Can you work these out from the model? Positions are in its coordinate system, mm. Round coordinates to 2 decimals unless told otherwise and drop trailing zeros. Loops run counter-clockwise (first coordinate to the right, second up) from the corner with the lowest first, then second, coordinate; pieces in that order, holes last. Notation, with made-up numbers: M 64,40.25 L 87,40.25 A22 cw 87,58.25 Z; hole C -19,78 d3. An arc over 180 degrees is marked long. Use a Markdown table: item, result. Add a question column.
```python
from build123d import *

# Parameters (mm, degrees)
SKETCH004_W  = 5.019769
SKETCH004_H  = 1.561025
PAD002_DEPTH = 1
PAD_DEPTH    = 0.5
PAD001_DEPTH = 0.5
PAD003_DEPTH = 0.5
PAD004_DEPTH = 0.5


with BuildPart() as part:
    # Sketch004 → Pad002 (new body)
    with BuildSketch(Plane.XZ.offset(1.25)):
        with Locations((1.436677, 3.083954)):
            Rectangle(SKETCH004_W, SKETCH004_H)
    extrude(amount=PAD002_DEPTH)

    # Sketch → Pad (join)
    with BuildSketch(Plane.YZ.offset(-0.75)):
        Polygon((-1.5, 3), (0.5, 3), (0.5, 17.5), (0, 17.5), (0, 3.5), (-1.5, 3.5), align=None)
    extrude(amount=PAD_DEPTH)

    # Sketch001 → Pad001 (join)
    with BuildSketch(Plane.YZ.offset(0.5)):
        Polygon((-1.5, 3), (0.5, 3), (0.5, 17.5), (0, 17.5), (0, 3.5), (-1.5, 3.5), align=None)
    extrude(amount=PAD001_DEPTH)

    # Sketch002 → Pad003 (join)
    with BuildSketch(Plane.YZ.offset(1.75)):
        Polygon((-1.5, 3), (0.5, 3), (0.5, 17.5), (0, 17.5), (0, 3.5), (-1.5, 3.5), align=None)
    extrude(amount=PAD003_DEPTH)

    # Sketch003 → Pad004 (join)
    with BuildSketch(Plane.YZ.offset(3)):
        Polygon((-1.5, 3), (0.5, 3), (0.5, 17.5), (0, 17.5), (0, 3.5), (-1.5, 3.5), align=None)
    extrude(amount=PAD004_DEPTH)


solid = part.part
```
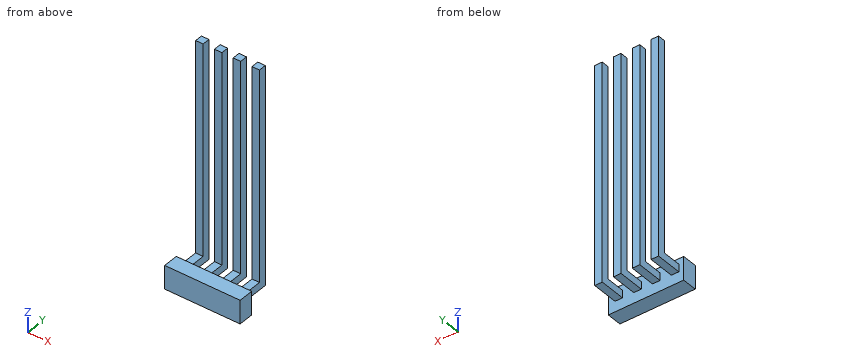
(1) I'm going to push flat-ended pins straight in: pin 1 (0.5 mm diameter, centred on y = 0, z = 11.5, fed in from +X); pin 2 (1 mm diameter, centred on x = 1.5, y = -0.5, fed in from +Z); pin 3 (0.6 mm diameter, centred on x = 1, y = -0.5, fed in from -Z). Where does each tip first touch, or does it pass through?
(2) Suppose I cut it at B-B on y = -0.25. List the corners of the cut face in (x, z) for me.
(3) Suppose I cut it at C-C on x = 0.7. List the corners of the cut face in (y, z) for me, and give its area (3 significant figures).
(4) Suppose I cut it at D-D on y = -1.8. List the corners of the cut face in (x, z) for me, and give its area (3 significant figures).
(5) Suppose I cut it at A-A on z = 7.5. List the corners of the cut face in (x, y) for me.
(6) If I drill on probe 1 along X at (y, z) = (0.1, 6.25); probe 2 along Z at (x, y) = (0.7, -1.6); probe 3 along Y at (x, z) = (-0.45, 8.75), over which ranges is the centre line in solid material (lowest first)? Write a range as [from, to].
Results below:
| question | item | result |
|---|---|---|
| 1 | pin 1 | stops at x = 3.5 |
| 1 | pin 2 | stops at z = 3.5 |
| 1 | pin 3 | stops at z = 3 |
| 2 | outline | M -0.75,3 L -0.25,3 L -0.25,3.5 L -0.75,3.5 Z; M 0.5,3 L 1,3 L 1,3.5 L 0.5,3.5 Z; M 1.75,3 L 2.25,3 L 2.25,3.5 L 1.75,3.5 Z; M 3,3 L 3.5,3 L 3.5,3.5 L 3,3.5 Z |
| 3 | outline | M -2.25,2.3 L -1.25,2.3 L -1.25,3 L 0.5,3 L 0.5,17.5 L 0,17.5 L 0,3.5 L -1.25,3.5 L -1.25,3.86 L -2.25,3.86 Z |
| 3 | area | 9.44 mm² |
| 4 | outline | M -1.07,2.3 L 3.95,2.3 L 3.95,3.86 L -1.07,3.86 Z |
| 4 | area | 7.84 mm² |
| 5 | outline | M -0.75,0 L -0.25,0 L -0.25,0.5 L -0.75,0.5 Z; M 0.5,0 L 1,0 L 1,0.5 L 0.5,0.5 Z; M 1.75,0 L 2.25,0 L 2.25,0.5 L 1.75,0.5 Z; M 3,0 L 3.5,0 L 3.5,0.5 L 3,0.5 Z |
| 6 | probe 1 | x = [-0.75, -0.25], [0.5, 1], [1.75, 2.25], [3, 3.5] |
| 6 | probe 2 | z = [2.3, 3.86] |
| 6 | probe 3 | y = [0, 0.5] |
